Work out the finished part from the listing and answer in its coordinate system (mm). A direction names the side the tool comes from. Round coordinates to 2 decimals unless told otherwise and drop trailing zeros. Order: outer loops, then holes, each group sorted by start corner. A loop starts at its lowest first (then second) coordinate and runs counter-clockwise, first axis right, second up.
Autodesk Fusion 360 part; units mm, degrees
sketch "Sketch1" plane through (0, 0, 0) normal (0, 0, 1) x (1, 0, 0)
  line L0 (3, 0) -> (61, 0)
  line L1 (64, 3) -> (64, 90)
  line L2 (61, 93) -> (3, 93)
  line L3 (0, 90) -> (0, 3)
  arc A0 (3, 93) -> (0, 90) centre (3, 90) ccw
  arc A1 (64, 90) -> (61, 93) centre (61, 90) ccw
  arc A2 (61, 0) -> (64, 3) centre (61, 3) ccw
  arc A3 (0, 3) -> (3, 0) centre (3, 3) ccw
  point P0 (64, 0)
  point P1 (0, 93)
  dimension "d1" = 64
  dimension "d2" = 93
  dimension "d3" = 3
  dimension "d4" = 3
extrude "Extrude1" add sketch "Sketch1" along normal blind 3
sketch "Sketch4" plane through (0, 0, 3) normal (0, 0, 1) x (-1, 0, 0)
  arc A0 (0, -3) -> (-3, 0) centre (-3, -3) ccw
  line L0 (-3, 0) -> (-61, 0)
  arc A1 (-61, 0) -> (-64, -3) centre (-61, -3) ccw
  line L1 (-64, -3) -> (-64, -90)
  arc A2 (-64, -90) -> (-61, -93) centre (-61, -90) ccw
  line L2 (-61, -93) -> (-3, -93)
  arc A3 (-3, -93) -> (0, -90) centre (-3, -90) ccw
  line L3 (0, -90) -> (0, -3)
  line L4 (-3, -3) -> (-61, -3)
  line L5 (-61, -3) -> (-61, -90)
  line L6 (-61, -90) -> (-3, -90)
  line L7 (-3, -90) -> (-3, -3)
  dimension "d11" = 58
  dimension "d12" = 87
  dimension "d13" = 3
  dimension "d14" = 3
extrude "Extrude2" add sketch "Sketch4" along normal blind 25
sketch "Sketch5" plane through (0, 0, 0) normal (0, -1, 0) x (1, 0, 0)
  line L0 (3, 0) -> (61, 0)
  line L1 (61, 0) -> (61, 23)
  line L2 (3, 23) -> (61, 23)
  line L3 (6, 6.8) -> (22.5, 6.8)
  line L4 (22.5, 6.8) -> (22.5, 23.8)
  line L5 (22.5, 23.8) -> (6, 23.8)
  line L6 (6, 23.8) -> (6, 6.8)
  line L7 (3, 0) -> (3, 23)
  line L8 (25.5, 23.8) -> (40.45, 23.8)
  line L9 (40.45, 23.8) -> (40.45, 6.8)
  line L10 (40.45, 6.8) -> (25.5, 6.8)
  line L11 (25.5, 6.8) -> (25.5, 23.8)
  line L12 (43.45, 6.8) -> (58.4, 6.8)
  line L13 (58.4, 6.8) -> (58.4, 23.8)
  line L14 (58.4, 23.8) -> (43.45, 23.8)
  line L15 (43.45, 23.8) -> (43.45, 6.8)
  line L16 (3, 0) -> (61, 0)
  line L17 (61, 0) -> (61, 28)
  line L18 (61, 28) -> (3, 28)
  line L19 (3, 28) -> (3, 0)
  dimension "d21" = 16.5
  dimension "d22" = 17
  dimension "d23" = 3
  dimension "d26" = 14.95
  dimension "d27" = 17
  dimension "d29" = 14.95
  dimension "d30" = 17
  dimension "d31" = 3
  dimension "d34" = 3
  dimension "d45" = 6.8
extrude "Extrude4" cut sketch "Sketch5" against normal blind 3 contours L2 L4 L5 L6 | L2 L3 L4 L6 | L2 L12 L13 L15 | L2 L13 L14 L15 | L2 L8 L9 L11 | L2 L9 L10 L11
sketch "Sketch6" plane through (0, 0, 3) normal (0, 0, 1) x (-1, 0, 0)
  line L0 (-3, -3) -> (-61, -3)
  line L1 (-61, -3) -> (-61, -90)
  line L2 (-61, -90) -> (-3, -90)
  line L3 (-3, -90) -> (-3, -3)
  circle A0 centre (-7.5, -85.5) radius 1
  circle A1 centre (-7.5, -85.5) radius 3
  circle A2 centre (-56.5, -85.5) radius 1
  circle A3 centre (-56.5, -85.5) radius 3
  circle A4 centre (-56.5, -27.5) radius 1
  circle A5 centre (-56.5, -27.5) radius 3
  circle A6 centre (-7.5, -27.5) radius 1
  circle A7 centre (-7.5, -27.5) radius 3
  dimension "d35" = 2
  dimension "d36" = 4.5
  dimension "d37" = 4.5
  dimension "d38" = 6
  dimension "d59" = 2
  dimension "d60" = 4.5
  dimension "d61" = 4.5
  dimension "d62" = 6
  dimension "d63" = 2
  dimension "d64" = 4.5
  dimension "d65" = 58
  dimension "d66" = 6
  dimension "d67" = 2
  dimension "d68" = 4.5
  dimension "d69" = 58
  dimension "d70" = 6
extrude "Extrude6" cut sketch "Sketch6" against normal blind 3 contours A0 | A2 | A4 | A6
extrude "Extrude7" add sketch "Sketch6" along normal blind 0.5 contours A1
sketch "Sketch7" plane through (0, 0, 0) normal (-1, 0, 0) x (0, -1, 0)
  line L0 (-90, 0) -> (-3, 0)
  line L1 (-3, 0) -> (-3, 28)
  line L2 (-3, 28) -> (-90, 28)
  line L3 (-90, 28) -> (-90, 0)
  line L4 (-88, 6) -> (-43, 6)
  line L5 (-43, 6) -> (-43, 11)
  line L6 (-43, 11) -> (-88, 11)
  line L7 (-88, 11) -> (-88, 6)
  dimension "d46" = 45
  dimension "d47" = 5
  dimension "d50" = 6
extrude "Extrude8" cut sketch "Sketch7" against normal blind 3 contours L4 L5 L6 L7
sketch "Sketch8" plane through (0, 93, 0) normal (0, 1, 0) x (-1, 0, 0)
  line L0 (-61, 0) -> (-3, 0)
  line L1 (-3, 0) -> (-3, 28)
  line L2 (-3, 28) -> (-61, 28)
  line L3 (-61, 28) -> (-61, 0)
  line L4 (-44.5, 3) -> (-19.5, 3)
  line L5 (-19.5, 3) -> (-19.5, 11)
  line L6 (-19.5, 11) -> (-44.5, 11)
  line L7 (-44.5, 11) -> (-44.5, 3)
  line L8 (-3, 0) -> (-3, 23)
  line L9 (-3, 0) -> (-61, 0)
  dimension "d51" = 25
  dimension "d52" = 8
  dimension "d53" = 16.5
  dimension "d54" = 3
extrude "Extrude9" cut sketch "Sketch8" against normal blind 3 contours L4 L5 L6 L7
extrude "Extrude10" add 1 faces at (9.6751, 86.3269, 3.5) along direction (0, 0, 1) blind 1.5
extrude "Extrude11" add sketch "Sketch6" along normal blind 2 contours A3 | A5 | A7
extrude "Extrude13" add sketch "Sketch6" along normal blind 3 contours A4
extrude "Extrude14" add sketch "Sketch6" along normal blind 3 contours A0 | A2 | A6
sketch "Sketch11" plane through (0, 0, 0) normal (-1, 0, 0) x (0, -1, 0)
  line L0 (-43, 6) -> (-88, 6)
  line L1 (-88, 6) -> (-88, 11)
  line L2 (-88, 11) -> (-43, 11)
  line L3 (-43, 11) -> (-43, 6)
  line L4 (-90, 0) -> (-3, 0)
  line L5 (-3, 0) -> (-3, 28)
  line L6 (-3, 28) -> (-90, 28)
  line L7 (-90, 28) -> (-90, 0)
  line L8 (-81.3, 28) -> (-59.3, 28)
  line L9 (-59.3, 28) -> (-59.3, 14.2)
  line L10 (-59.3, 14.2) -> (-81.3, 14.2)
  line L11 (-81.3, 14.2) -> (-81.3, 28)
  dimension "d85" = 22
  dimension "d86" = 13.8
  dimension "d87" = 8.7
extrude "Extrude15" cut sketch "Sketch11" against normal blind 3 contours L6 L8 L9 L10 L11
fillet "Fillet1" radius 1 1 edges at (1.5, 81.3, 14.2)
fillet "Fillet2" radius 1 21 edges at (1.5, 59.3, 14.2) (44.5, 91.5, 3) (44.5, 91.5, 11) (19.5, 91.5, 3) (19.5, 91.5, 11) (1.5, 43, 6) (6, 1.5, 6.8) (25.5, 1.5, 6.8) (43.45, 1.5, 6.8) (6, 1.5, 23.8) (25.5, 1.5, 23.8) (43.45, 1.5, 23.8) (40.45, 1.5, 23.8) (22.5, 1.5, 23.8) (58.4, 1.5, 23.8) (1.5, 88, 11) (1.5, 88, 6) (22.5, 1.5, 6.8) (40.45, 1.5, 6.8) (58.4, 1.5, 6.8) (1.5, 43, 11)
delete_face "DeleteFace1" 1 faces at (1, 80.5358, 14.2282)
delete_face "DeleteFace2" 1 faces at (1, 59.4854, 14.6199)
Item 1: Find the intervals of material crossed by line 1 along Y through (x, z) = (7.5, 1.7); line 2 along X through (y, z) = (27.5, 1.45); line 3 along Y through (x, z) = (17, 3.5), in increasing order.
Item 2: Given pin 1 (2 mm diameter, centred on x = 22, z = 21.5, fed in from -Y); pin 2 (1 mm diameter, centred on x = 8, y = 28, fed in from +Z); pin 3 (6 mm diameter, centred on x = 29, z = 10.5, fed in from -Y); pin 4 (4 mm diameter, centred on x = 19.5, y = 50, fed in from +Z), each flat-ended and moving along its own axis, determine where each tip first touches the part or whether it passes through.
Item 3: For a pull along Y with two mould halves and no side action, classify faces 1 (the face through (57, 27, 6)), 2 (the face through (33, 1, 23.8)), 3 (the face through (25, 0, 11)) as released by +Y, released by -Y, zero draft, split by the parting line, or undercut.
Item 4: Find section B-B (z = 21.75). Write down the section's boundary in (x, y).
Item 5: Find section D-D (z = 8.75). State how many separate pieces and enclosed holes the cut face has, plus the area to 3 significant figures.
Item 6: Find section A-A (x = 28). Write down the section's boundary in (y, z).
Item 7: Find section C-C (x = 12). Write down the section's boundary in (y, z), plus the area to 3 significant figures.
Item 8: A tool of negligible diameter and unlimited length cuts with its end or side. For faces 4 (the face through (32, 47, 0)), 5 (the face through (1, 70, 14.2)), 6 (the face through (7.63, 26.51, 1.52)), 7 (the face through (51, 1, 6.8)), 8 (the face through (55, 85, 5)), from which of +Z, -Z, +X, -X, +Y, -Y can it reach the whole face along a straight path? Write none if from no direction.
Model answer:
1. line 1: y = 0 to 26.5, 28.5 to 84.5, 86.5 to 93
1. line 2: x = 0 to 6.5, 8.5 to 55.5, 57.5 to 64
1. line 3: y = 0 to 3, 90 to 93
2. pin 1: stops at y = 0
2. pin 2: stops at z = 6
2. pin 3: stops at y = 90
2. pin 4: stops at z = 3
3. face 1: undercut
3. face 2: zero draft
3. face 3: released by -Y
4. outline: (0, 3) arc R3 ccw to (3, 0) - (6, 0) - (6, 3) - (3, 3) - (3, 59.3) - (0, 59.3) - close; (0, 81.3) - (3, 81.3) - (3, 90) - (61, 90) - (61, 3) - (58.4, 3) - (58.4, 0) - (61, 0) arc R3 ccw to (64, 3) - (64, 90) arc R3 ccw to (61, 93) - (3, 93) arc R3 ccw to (0, 90) - close; (22.5, 0) - (25.5, 0) - (25.5, 3) - (22.5, 3) - close; (40.45, 0) - (43.45, 0) - (43.45, 3) - (40.45, 3) - close
5. separate pieces: 5
5. enclosed holes: 0
5. area: 549 mm2
6. outline: (0, 0) - (93, 0) - (93, 3) - (3, 3) - (3, 6.8) - (0, 6.8) - close; (0, 23.8) - (3, 23.8) - (3, 28) - (0, 28) - close; (90, 11) - (93, 11) - (93, 28) - (90, 28) - close
7. outline: (0, 0) - (93, 0) - (93, 28) - (90, 28) - (90, 3) - (3, 3) - (3, 6.8) - (0, 6.8) - close; (0, 23.8) - (3, 23.8) - (3, 28) - (0, 28) - close
7. area: 378 mm2
8. face 4: -Z, +X, -X, +Y, -Y
8. face 5: +Z, -X
8. face 6: -Z
8. face 7: -Y
8. face 8: +Z
